from build123d import *

# Parameters (mm, degrees)
DODANIE_WYCI_GNI_CIE1_DEPTH = 1
SZKIC2_R                    = 3.15
WYTNIJ_WYCI_GNI_CIE1_DEPTH  = 1


with BuildPart() as part:
    # Szkic1 → Dodanie-wyciągnięcie1 (new body)
    with BuildSketch(Plane.XY):
        with BuildLine():
            Line((-12.5, -6), (-12.5, -16))
            Line((-12.5, -16), (12.5, -16))
            Line((12.5, -16), (12.5, -6))
            Line((12.5, -6), (7.91, -6))
            ThreePointArc((7.91, -6), (6.495786438, -5.414213562), (5.91, -4))
            Line((5.91, -4), (5.91, 5.45))
            Line((5.91, 5.45), (5.91, 6.85))
            Line((5.91, 6.85), (5.91, 10.85))
            Line((5.91, 10.85), (-5.85, 10.85))
            Line((-5.85, 10.85), (-5.85, 6.85))
            Line((-5.85, 6.85), (-5.85, 5.45))
            Line((-5.85, 5.45), (-5.85, -4))
            ThreePointArc((-5.85, -4), (-6.435786438, -5.414213562), (-7.85, -6))
            Line((-7.85, -6), (-12.5, -6))
        make_face()
    extrude(amount=DODANIE_WYCI_GNI_CIE1_DEPTH)

    # Szkic2 → Wytnij-wyciągnięcie1 (cut)
    with BuildSketch(Plane.XY.offset(1)):
        with Locations((0.03, 5.36)):
            Circle(SZKIC2_R)
    extrude(amount=-WYTNIJ_WYCI_GNI_CIE1_DEPTH, mode=Mode.SUBTRACT)


solid = part.part
Could you check a few things on this model? Use its own coordinates, in mm. A direction names the side the tool comes from. Give positions to 0.01 mm unless a question says otherwise; leave off trailing zeros. Order: outer loops, then holes, each group sorted by start corner. A loop starts at its lowest first (then second) coordinate and runs counter-clockwise, first axis right, second up. Notation, with made-up numbers: (38, -4) -> (75, -4) arc R22 cw to (75, 25) -> close; hole circle Ø10 at (-3.75, 87.5). An arc over 180 degrees is marked (long way). Return JSON: item names as keys, results as strings.
1. Imagine slicing it at C-C on y = 5.36. List the corners of the cut face in (x, z) for me.
Answer list:
{"outline": "(-5.85, 0) -> (-3.12, 0) -> (-3.12, 1) -> (-5.85, 1) -> close; (3.18, 0) -> (5.91, 0) -> (5.91, 1) -> (3.18, 1) -> close"}
2. I need wall thicknesses on line 1 (Y direction, x = 0.03, z = 0.75); line 2 (X direction, y = -2.75, z = 0.95); line 3 (Y direction, x = 10.5, z = 0.4). Which ranges of each line are inside material? Lowest first, please. Write a range as from..to.
Answer list:
{"line 1": "y = -16..2.21, 8.51..10.85", "line 2": "x = -5.85..5.91", "line 3": "y = -16..-6"}
3. Imagine slicing it at A-A on x = 0.03. List the corners of the cut face in (y, z) for me.
Answer list:
{"outline": "(-16, 0) -> (2.21, 0) -> (2.21, 1) -> (-16, 1) -> close; (8.51, 0) -> (10.85, 0) -> (10.85, 1) -> (8.51, 1) -> close"}
4. Imagine slicing it at D-D on y = -1.75. List the corners of the cut face in (x, z) for me, then the cut area to 3 significant figures.
Answer list:
{"outline": "(-5.85, 0) -> (5.91, 0) -> (5.91, 1) -> (-5.85, 1) -> close", "area": "11.8 mm2"}
5. On a 3-axis mill with a long thin cutter (end or side, diameter ignored), from which of +Z, -Z, +X, -X, +Y, -Y can I reach the whole of each face in a straight line? I mean faces 5 (the flat face through (-12.5, -10.9, 0.5)), 6 (the flat face through (10.2, -6, 0.5)), 7 (the flat face through (-10.1, -6, 0.5)). Say none if no direction works.
Answer list:
{"face 5": "+Z, -Z, -X, +Y, -Y", "face 6": "+Z, -Z, +X, +Y", "face 7": "+Z, -Z, -X, +Y"}
6. Imagine slicing it at B-B on z = 0.6. List the corners of the cut face in (x, y) for me.
Answer list:
{"outline": "(-12.5, -16) -> (12.5, -16) -> (12.5, -6) -> (7.91, -6) arc R2 cw to (5.91, -4) -> (5.91, 10.85) -> (-5.85, 10.85) -> (-5.85, -4) arc R2 cw to (-7.85, -6) -> (-12.5, -6) -> close; hole circle Ø6.3 at (0.03, 5.36)"}
7. Thinking about a two-plate mould opening in Y: for faces 1 (the flat face through (-5.85, 3.5, 0.5)), 2 (the cylindrical face through (-0.38, 8.483, 0.507)), 3 (the flat face through (0.1, 10.85, 0.5)), 4 (the flat face through (-0.2, -16, 0.5)), which applies, pulls with the +Y half, pulls with the -Y half, needs draft (parallel to the pull), parting line crosses it, or undercut?
Answer list:
{"face 1": "needs draft", "face 2": "undercut", "face 3": "pulls with the +Y half", "face 4": "pulls with the -Y half"}
